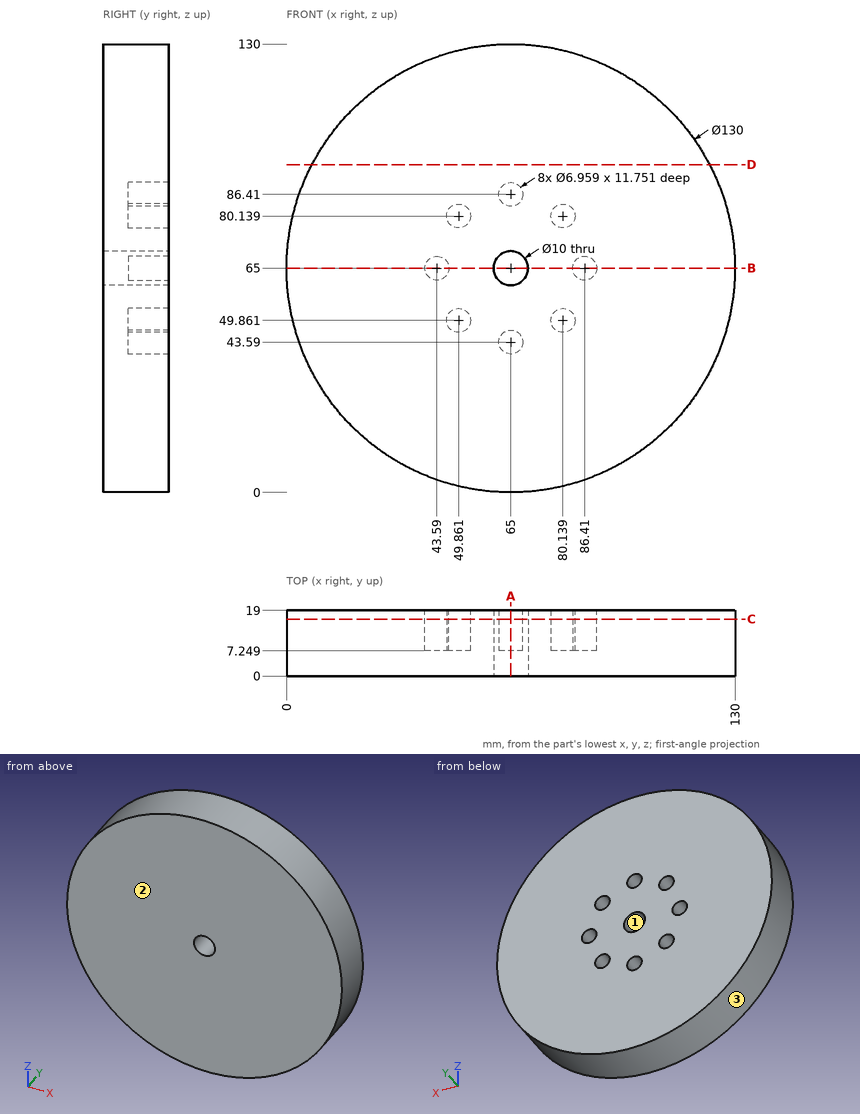
Check sheet for the drawn part. Datum: minimum x, y, z corner. Units: mm. Coordinates: 2 decimals unless noted, no trailing zeros. Order: outer loops, then holes, each group sorted by start corner. A loop starts at its lowest first (then second) coordinate and runs counter-clockwise, first axis right, second up. Notation, with made-up numbers: (61, -18) -> (86, -18) arc R24 ccw to (86, 16) -> close; hole circle Ø4 at (63.25, 70). An arc over 180 degrees is marked (long way). Use a Markdown table: item, result. Add a question column.
1. Cross-section at B-B (z = 65). Enter the section's corners in (x, y), and give its area (3 significant figures).
2. Material ranges on L1, parallel to X at y = 14.5, z = 65; L2, parallel to Z at x = 88, y = 10.25 (1 decimal); L3, parallel to X at y = 4.5, z = 60.5 (1 decimal), recorded low to high.
3. Cross-section at C-C (y = 16.5). Give the number of separate pieces and of enclosed holes in the cut face, and give its area (3 significant figures).
4. Go/stop test with flat-tipped pins: pin 1 Ø8 at (x, y) = (30, 11.5) entering from +Z; pin 2 Ø2 at (y, z) = (9.5, 86.5) entering from +X; pin 3 Ø2 at (x, z) = (65.5, 43.5) entering from +Y. Record where each tip stops, or that it passes through.
5. Mould release check, pull along X, two halves, no side actions. Record for the marked faces 1, 2 and 3: pulls with the +X half, pulls with the -X half, needs draft (parallel to the pull), parting line crosses it, or undercut.
6. Cross-section at D-D (z = 95). Enter the section's corners in (x, y), and give its area (3 significant figures).
7. Cross-section at A-A (x = 65). Enter the section's corners in (y, z), and give its area (3 significant figures).
Filled sheet:
| question | item | result |
|---|---|---|
| 1 | outline | (0, 0) -> (60, 0) -> (60, 19) -> (47.07, 19) -> (47.07, 7.25) -> (40.11, 7.25) -> (40.11, 19) -> (0, 19) -> close; (70, 0) -> (130, 0) -> (130, 19) -> (89.89, 19) -> (89.89, 7.25) -> (82.93, 7.25) -> (82.93, 19) -> (70, 19) -> close |
| 1 | area | 2,120 mm2 |
| 2 | L1 | 0 to 40.11, 47.07 to 60, 70 to 82.93, 89.89 to 130 |
| 2 | L2 | 4.2 to 61.9, 68.1 to 125.8 |
| 2 | L3 | 0.2 to 62.8, 67.2 to 129.8 |
| 3 | separate pieces | 1 |
| 3 | enclosed holes | 9 |
| 3 | area | 12,900 mm2 |
| 4 | pin 1 | z = 122.13 |
| 4 | pin 2 | x = 126.68 |
| 4 | pin 3 | y = 7.25 |
| 5 | face 1 | undercut |
| 5 | face 2 | needs draft |
| 5 | face 3 | parting line crosses it |
| 6 | outline | (7.34, 0) -> (122.66, 0) -> (122.66, 19) -> (7.34, 19) -> close |
| 6 | area | 2,190 mm2 |
| 7 | outline | (0, 0) -> (19, 0) -> (19, 40.11) -> (7.25, 40.11) -> (7.25, 47.07) -> (19, 47.07) -> (19, 60) -> (0, 60) -> close; (0, 70) -> (19, 70) -> (19, 82.93) -> (7.25, 82.93) -> (7.25, 89.89) -> (19, 89.89) -> (19, 130) -> (0, 130) -> close |
| 7 | area | 2,120 mm2 |
